Design review of the part built by this model. Coordinates are the model's own, in mm. A direction names the side the tool comes from. Coordinates: 2 decimals unless noted, no trailing zeros. Write each loop counter-clockwise with the first axis right and the second up, starting at its lowest first coordinate (ties: lowest second). Pieces come first, ordered by that corner, then holes. Notation, with made-up numbers: (2.25, 81) - (30.25, 81) arc R32 ccw to (30.25, 120) - close; hole circle Ø1 at (40, -38). An arc over 180 degrees is marked (long way). One line per item, written item: value.
from build123d import *

# Parameters (mm, degrees)
SKETCH1_W           = 88.9
SKETCH1_H           = 152.4
SKETCH1_W_2         = 12.7
SKETCH1_H_2         = 50.8
SKETCH1_W_3         = 6.477
SKETCH1_H_3         = 12.954
BOSS_EXTRUDE1_DEPTH = 6.35
SKETCH3_W           = 6.477
SKETCH3_H           = 12.827
SKETCH3_R           = 1.651
CUT_EXTRUDE3_DEPTH  = 6.35
SKETCH4_R           = 1.651
CUT_EXTRUDE4_DEPTH  = 6.35
FILLET1_R           = 2.54
SKETCH5_R           = 1.905
CUT_EXTRUDE5_DEPTH  = 6.35


with BuildPart() as part:
    # Sketch1 → Boss-Extrude1 (new body)
    # profile 1 of 2: a face of its own
    with BuildSketch(Plane.XY):
        with Locations((44.45, 76.2)):
            Rectangle(SKETCH1_W, SKETCH1_H)
    # profile 2 of 2: a face of its own
    with BuildSketch(Plane.XY):
        with Locations((58.963500056, -25.4)):
            Rectangle(SKETCH1_W_2, SKETCH1_H_2)
        with Locations((58.963500056, -41.402)):
            Rectangle(SKETCH1_W_3, SKETCH1_H_3, mode=Mode.SUBTRACT)
        with Locations((58.963500056, -9.398)):
            Rectangle(SKETCH1_W_3, SKETCH1_H_3, mode=Mode.SUBTRACT)
    extrude(amount=BOSS_EXTRUDE1_DEPTH)

    # Sketch3 → Cut-Extrude3 (cut)
    with BuildSketch(Plane.XY.offset(6.35)):
        with Locations((6.4135, 139.6365)):
            Rectangle(SKETCH3_W, SKETCH3_H)
        with Locations((6.4135, 12.7635)):
            Rectangle(SKETCH3_W, SKETCH3_H)
        with Locations((82.4865, 139.6365)):
            Rectangle(SKETCH3_W, SKETCH3_H)
        with Locations((6.4135, 120.523)):
            Circle(SKETCH3_R)
        with Locations((6.4135, 76.2)):
            Rectangle(SKETCH3_W, SKETCH3_H)
        with Locations((6.4135, 31.877)):
            Circle(SKETCH3_R)
        with Locations((82.4865, 12.7635)):
            Rectangle(SKETCH3_W, SKETCH3_H)
        with Locations(Location((82.4865, 31.877, 0), (0, 0, 180))):
            Circle(SKETCH3_R)
        with Locations(Location((82.4865, 120.523, 0), (0, 0, 180))):
            Circle(SKETCH3_R)
        with Locations((82.4865, 76.2)):
            Rectangle(SKETCH3_W, SKETCH3_H)
    extrude(amount=-CUT_EXTRUDE3_DEPTH, mode=Mode.SUBTRACT)

    # Sketch4 → Cut-Extrude4 (cut)
    with BuildSketch(Plane.XY.offset(6.35)):
        with Locations((58.963500056, -19.05)):
            Circle(SKETCH4_R)
        with Locations((58.963500056, -31.75)):
            Circle(SKETCH4_R)
    extrude(amount=-CUT_EXTRUDE4_DEPTH, mode=Mode.SUBTRACT)

    # Fillet1
    fillet1_edges = [part.edges().sort_by_distance(p)[0] for p in [
        (0, 0, 3.175),
        (0, 152.4, 3.175),
        (88.9, 152.4, 3.175),
        (88.9, 0, 3.175),
        (65.313500056, 0, 3.175),
        (65.313500056, -50.8, 3.175),
        (52.613500056, -50.8, 3.175),
        (52.613500056, 0, 3.175),
    ]]
    fillet(fillet1_edges, radius=FILLET1_R)

    # Sketch5 → Cut-Extrude5 (cut)
    with BuildSketch(Plane.XY.offset(6.35)):
        with Locations((63.5, 139.7)):
            Circle(SKETCH5_R)
        with Locations((63.5, 101.6)):
            Circle(SKETCH5_R)
    extrude(amount=-CUT_EXTRUDE5_DEPTH, mode=Mode.SUBTRACT)


solid = part.part
1. Wall thickness on line 1 along Y through (x, z) = (56, 3.5) (3 decimals); line 2 along Y through (x, z) = (85.5, 3.25); line 3 along X through (y, z) = (-13.5, 5.25) (1 decimal): over which ranges is each line inside the solid? List them lowest first.
Answer block:
line 1: y = -50.8 to -47.879, -34.925 to -15.875, -2.921 to 152.4
line 2: y = 0 to 6.35, 19.18 to 69.79, 82.61 to 133.22, 146.05 to 152.4
line 3: x = 52.6 to 55.7, 62.2 to 65.3
2. Insertion check: pin 1 Ø3.5 at (x, y) = (63.5, 101.6) entering from +Z; pin 2 Ø1.9 at (y, z) = (-39.5, 4.5) entering from -X. Each pin has a flat end and moves straight along its axis. Give the tip position at first contact, or say it passes through.
Answer block:
pin 1: passes through
pin 2: stops at x = 52.61
3. Consider section B-B, the plane y = 101.6. Write out the cut boundary in (x, z) (3 decimals).
Answer block:
outline: (0, 0) - (61.595, 0) - (61.595, 6.35) - (0, 6.35) - close; (65.405, 0) - (88.9, 0) - (88.9, 6.35) - (65.405, 6.35) - close
4. Mouldability with a two-part tool opening along X and no side actions: class faces 3 (the face through (65.314, -26, 3)), 4 (the face through (82, 133.223, 3)), 5 (the face through (26, 0, 3)) as released by +X, released by -X, zero draft, split by the parting line, or undercut.
Answer block:
face 3: released by +X
face 4: undercut
face 5: zero draft
5. Consider section C-C, the plane x = 20. Write out the cut boundary in (y, z).
Answer block:
outline: (0, 0) - (152.4, 0) - (152.4, 6.35) - (0, 6.35) - close
6. Consider section A-A, the plane y = 139.7. Write out the cut boundary in (x, z) (3 decimals), then the cut area to 3 significant figures.
Answer block:
outline: (0, 0) - (3.175, 0) - (3.175, 6.35) - (0, 6.35) - close; (9.652, 0) - (61.595, 0) - (61.595, 6.35) - (9.652, 6.35) - close; (65.405, 0) - (79.248, 0) - (79.248, 6.35) - (65.405, 6.35) - close; (85.725, 0) - (88.9, 0) - (88.9, 6.35) - (85.725, 6.35) - close
area: 458 mm^2
7. For faces 1 (the face through (44, 152.4, 3)), 2 (the face through (55.725, -9, 3)), list the 3-axis set-ups (+Z, -Z, +X, -X, +Y, -Y) from which the entire face can be reached by the end or side of a thin tool; tool diameter is ignored.
Answer block:
face 1: +Z, -Z, +X, -X, +Y
face 2: +Z, -Z
